Here's how the part is built. I have some questions about the finished solid (model axes, mm). A direction names the side the tool comes from. Coordinates: 2 decimals unless noted, no trailing zeros. Loops run counter-clockwise (first coordinate to the right, second up) from the corner with the lowest first, then second, coordinate; pieces in that order, holes last.
from build123d import *

# Parameters (mm, degrees)
BOSS_EXTRUDE1_DEPTH = 2
SKETCH2_R           = 1.05
BOSS_EXTRUDE2_DEPTH = 2.6
SKETCH3_W           = 3
SKETCH3_H           = 5
BOSS_EXTRUDE3_DEPTH = 5
SKETCH4_W           = 2
SKETCH4_H           = 4
CUT_EXTRUDE1_DEPTH  = 24.631588809
FILLET1_R           = 0.5
FILLET2_R           = 0.2


with BuildPart() as part:
    # Sketch1 → Boss-Extrude1 (new body)
    with BuildSketch(Plane(origin=(0, 0, 0), x_dir=(0, 0, -1), z_dir=(1, 0, 0))):
        with BuildLine():
            Line((-17.23490614, 15.515536013), (-17.23490614, -2.484463987))
            ThreePointArc((-17.23490614, -2.484463987), (-14.73490614, -4.984463987), (-12.23490614, -2.484463987))
            Line((-12.23490614, -2.484463987), (-12.23490614, 15.515536013))
            ThreePointArc((-12.23490614, 15.515536013), (-14.73490614, 18.015536013), (-17.23490614, 15.515536013))
        make_face()
    extrude(amount=BOSS_EXTRUDE1_DEPTH)

    # Sketch2 → Boss-Extrude2 (add)
    with BuildSketch(Plane(origin=(2, 0, 0), x_dir=(0, 0, -1), z_dir=(1, 0, 0))):
        with Locations(Location((-14.73490614, 15.515536013, 0), (0, 0, 180))):
            Circle(SKETCH2_R)
    extrude(amount=BOSS_EXTRUDE2_DEPTH)

    # Sketch3 → Boss-Extrude3 (add)
    with BuildSketch(Plane(origin=(0, 0, 12.23490614), x_dir=(-1, 0, 0), z_dir=(0, 0, -1))):
        with Locations((1.5, 8.015536013)):
            Rectangle(SKETCH3_W, SKETCH3_H)
    extrude(amount=-BOSS_EXTRUDE3_DEPTH)

    # Sketch4 → Cut-Extrude1 (cut, through all)
    with BuildSketch(Plane(origin=(0, 10.515536013, 0), x_dir=(1, 0, 0), z_dir=(0, 1, 0))):
        with Locations((-1.5, -14.73490614)):
            Rectangle(SKETCH4_W, SKETCH4_H)
    extrude(amount=-CUT_EXTRUDE1_DEPTH, mode=Mode.SUBTRACT)

    # Fillet1
    fillet1_edges = [part.edges().sort_by_distance(p)[0] for p in [
        (-3, 8.015536013, 12.23490614),
        (-3, 8.015536013, 17.23490614),
    ]]
    fillet(fillet1_edges, radius=FILLET1_R)

    # Fillet2
    fillet2_edges = [part.edges().sort_by_distance(p)[0] for p in [
        (-1.5, 5.515536013, 12.73490614),
        (-2.5, 5.515536013, 14.73490614),
        (-1.5, 5.515536013, 16.73490614),
        (-0.5, 5.515536013, 14.73490614),
        (-0.5, 10.515536013, 14.73490614),
        (-1.5, 10.515536013, 12.73490614),
        (-2.5, 10.515536013, 14.73490614),
        (-1.5, 10.515536013, 16.73490614),
    ]]
    fillet(fillet2_edges, radius=FILLET2_R)


solid = part.part
Q1. For faces 1 (the flat face through (0, 0, 15)), 2 (the cylindrical face through (3.282, 14.474, 14.598)), 3 (the flat face through (-2, 8, 12.735)), 4 (the flat face through (1, 7, 17.235)), which set-ups out of +Z, -Z, +X, -X, +Y, -Y let a thin tool reach every point of the face, with its end or its side?
Q2. Suppose I cut it at D-D on z = 14.85. Write out the boundary of the cut face in (x, y), and give its area (3 significant figures).
Q3. Please list where these lines run through material, in increasing order: probe 1 along Z at (x, y) = (-1.75, 7); probe 2 along X at (y, z) = (4, 14.55); probe 3 along X at (y, z) = (6, 14.05).
Q4. Suppose I cut it at A-A on x = -1. Write out the boundary of the cut face in (y, z), and give its area (3 significant figures).
Q5. Suppose I cut it at C-C on y = 6.5. Write out the boundary of the cut face in (x, z).
Q6. Suppose I cut it at B-B on z = 13. Write out the boundary of the cut face in (x, y), and give its area (3 significant figures).
Q7. Will these pins go through, and if not, where does the flat tip stop? P1, Ø1.5, axis at y = 1.5, z = 16, coming from the +X side; P2, Ø1.5, axis at x = -2, z = 15, coming from the +Y side; P3, Ø1.5, axis at y = 1, z = 13.5, coming from the -X side.
Q8. We'd pull the mould along X, two halves only. Please class faces 5 (the flat face through (-2, 8, 16.735)), 6 (the flat face through (0, 14, 15)), 7 (the flat face through (0, 6, 12.235)), 8 (the flat face through (4.6, 16, 15)): pulls with the +X half, pulls with the -X half, needs draft (parallel to the pull), parting line crosses it, or undercut.
Check values:
1. face 1: +Z, -Z, -X, -Y
1. face 2: +X
1. face 3: +Y, -Y
1. face 4: +Z, +X, -X, +Y, -Y
2. outline: (-3, 5.52) - (-2.7, 5.52) arc R0.2 ccw to (-2.5, 5.72) - (-2.5, 10.32) arc R0.2 ccw to (-2.7, 10.52) - (-3, 10.52) - close; (-0.5, 5.72) arc R0.2 ccw to (-0.3, 5.52) - (0, 5.52) - (0, -4.98) - (2, -4.98) - (2, 14.47) - (4.6, 14.47) - (4.6, 16.56) - (2, 16.56) - (2, 18.01) - (0, 18.01) - (0, 10.52) - (-0.3, 10.52) arc R0.2 ccw to (-0.5, 10.32) - close
2. area: 56.4 mm2
3. probe 1: z = 12.23 to 12.73, 16.73 to 17.23
3. probe 2: x = 0 to 2
3. probe 3: x = -3 to -2.5, -0.5 to 2
4. outline: (5.52, 12.23) - (10.52, 12.23) - (10.52, 12.53) arc R0.2 ccw to (10.32, 12.73) - (5.72, 12.73) arc R0.2 ccw to (5.52, 12.53) - close; (5.52, 16.93) arc R0.2 ccw to (5.72, 16.73) - (10.32, 16.73) arc R0.2 ccw to (10.52, 16.93) - (10.52, 17.23) - (5.52, 17.23) - close
4. area: 4.97 mm2
5. outline: (-3, 12.73) arc R0.5 ccw to (-2.5, 12.23) - (2, 12.23) - (2, 17.23) - (-2.5, 17.23) arc R0.5 ccw to (-3, 16.73) - close; hole (-2.5, 12.73) - (-0.5, 12.73) - (-0.5, 16.73) - (-2.5, 16.73) - close
6. outline: (-3, 5.52) - (-2.7, 5.52) arc R0.2 ccw to (-2.5, 5.72) - (-2.5, 10.32) arc R0.2 ccw to (-2.7, 10.52) - (-3, 10.52) - close; (-0.5, 5.72) arc R0.2 ccw to (-0.3, 5.52) - (0, 5.52) - (0, -4.28) - (2, -4.28) - (2, 17.32) - (0, 17.32) - (0, 10.52) - (-0.3, 10.52) arc R0.2 ccw to (-0.5, 10.32) - close
6. area: 48.2 mm2
7. P1: stops at x = 2
7. P2: stops at y = 10.52
7. P3: stops at x = 0
8. face 5: undercut
8. face 6: pulls with the -X half
8. face 7: needs draft
8. face 8: pulls with the +X half
